Verification items for this drawing (mm, ordinates from the low corner). A direction names the side the tool comes from. Coordinates: 2 decimals unless noted, no trailing zeros. Order: outer loops, then holes, each group sorted by start corner. A loop starts at its lowest first (then second) coordinate and runs counter-clockwise, first axis right, second up. Notation, with made-up numbers: (84.5, 62) -> (113.5, 62) arc R16 ccw to (113.5, 87) -> close; hole circle Ø7 at (75.5, 5). An arc over 180 degrees is marked (long way). Answer in a Markdown table with one row per item. Add a question column.
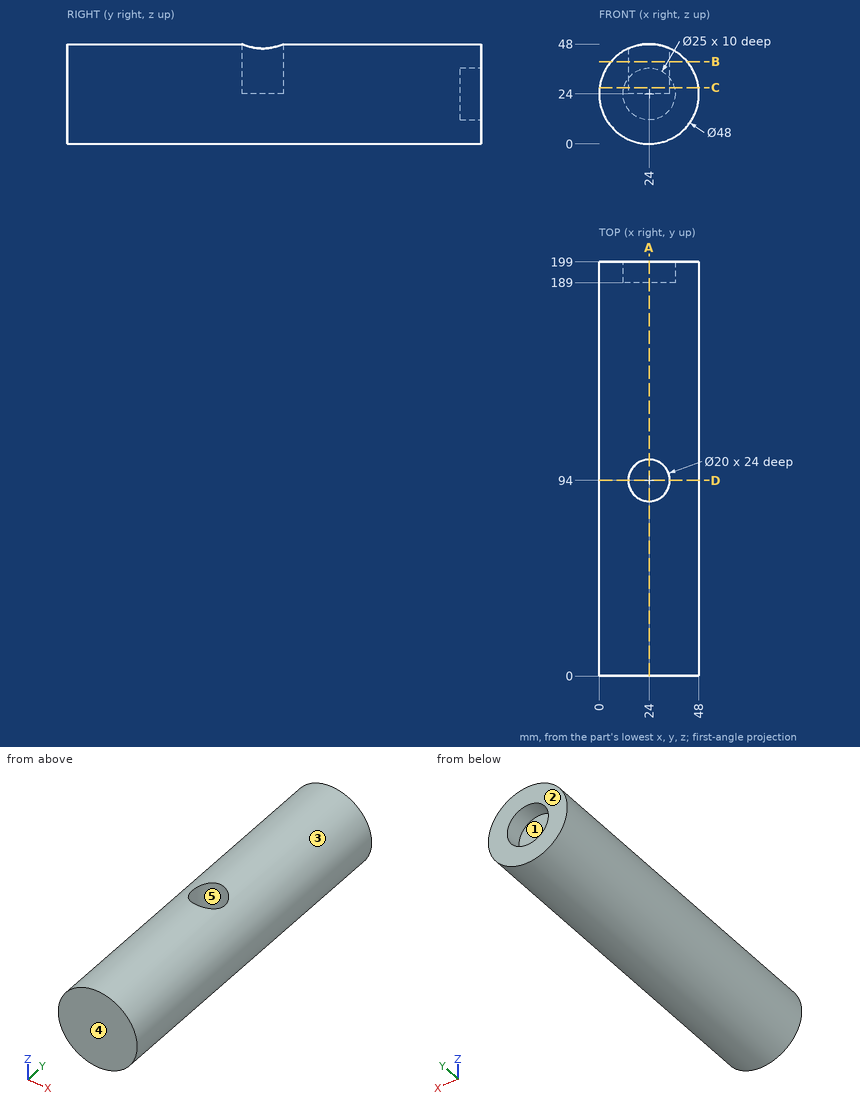
(1) Cross-section at B-B (z = 39.5). Enter the section's corners in (x, y).
(2) Access from +Z, -Z, +X, -X, +Y, -Y to the whole of each face (thin tool, end or side, straight path). Record for the marked faces 1 and 2.
(3) Cross-section at D-D (y = 94). Enter the section's corners in (x, z).
(4) Go/stop test with flat-tipped pins: P1, Ø1, axis at y = 32.5, z = 26.5, coming from the -X side; P2, Ø1, axis at y = 91, z = 20.5, coming from the +X side; P3, Ø6, axis at x = 6, y = 158.5, coming from the -Z side (3 decimals). Record where each tip stops, or that it passes through.
(5) Mould release check, pull along Y, two halves, no side actions. Record for the marked faces 3, 4 and 5: +Y half, -Y half, draft (parallel to the pull), parting line (faces both ways), or undercut.
(6) Scan lines: line 1 along Z through (x, y) = (24, 196); line 2 along Y through (x, z) = (24, 38); line 3 along Y through (x, z) = (24, 32.5). Record each from-to range of solid material in increasing order.
(7) Cross-section at A-A (x = 24). Enter the section's corners in (y, z).
(8) Cross-section at C-C (z = 27). Enter the section's corners in (x, y), plus the area to 3 significant figures.
Checks:
| question | item | result |
|---|---|---|
| 1 | outline | (5.68, 0) -> (42.32, 0) -> (42.32, 199) -> (5.68, 199) -> close; hole circle Ø20 at (24, 94) |
| 2 | face 1 | +Y |
| 2 | face 2 | +Z, -Z, +X, -X, +Y |
| 3 | outline | (14, 24) -> (14, 45.82) arc R24 ccw (long way) to (34, 45.82) -> (34, 24) -> close |
| 4 | P1 | x = 0.08 |
| 4 | P2 | x = 47.81 |
| 4 | P3 | z = 5.265 |
| 5 | face 3 | draft |
| 5 | face 4 | -Y half |
| 5 | face 5 | undercut |
| 6 | line 1 | 0 to 11.5, 36.5 to 48 |
| 6 | line 2 | 0 to 84, 104 to 199 |
| 6 | line 3 | 0 to 84, 104 to 189 |
| 7 | outline | (0, 0) -> (199, 0) -> (199, 11.5) -> (189, 11.5) -> (189, 36.5) -> (199, 36.5) -> (199, 48) -> (104, 48) -> (104, 24) -> (84, 24) -> (84, 48) -> (0, 48) -> close |
| 8 | outline | (0.19, 0) -> (47.81, 0) -> (47.81, 199) -> (36.13, 199) -> (36.13, 189) -> (11.87, 189) -> (11.87, 199) -> (0.19, 199) -> close; hole circle Ø20 at (24, 94) |
| 8 | area | 8,920 mm² |
